```python
from build123d import *

# Parameters (mm, degrees)
SKETCH1_R           = 25
SKETCH1_W           = 27.8
SKETCH1_H           = 27.8
BOSS_EXTRUDE1_DEPTH = 55
BOSS_EXTRUDE2_START = 5
SKETCH2_R           = 25
SKETCH2_W           = 27.8
SKETCH2_H           = 27.8
BOSS_EXTRUDE2_DEPTH = 5
SKETCH3_W           = 25
SKETCH3_H           = 50
BOSS_EXTRUDE3_DEPTH = 80
FILLET1_R           = 2.5
FILLET2_R           = 2.5
SKETCH21_W          = 60
SKETCH21_H          = 20.6
CUT_EXTRUDE1_DEPTH  = 11.3
SKETCH22_W          = 40.5
SKETCH22_H          = 20.6
CUT_EXTRUDE2_DEPTH  = 93.059763198
CUT_EXTRUDE3_DEPTH  = 88.464278423
SKETCH23_R          = 2.15
CUT_EXTRUDE4_DEPTH  = 93.059763198
CUT_EXTRUDE7_DEPTH  = 27.5
CUT_EXTRUDE8_DEPTH  = 10


with BuildPart() as part:
    # Sketch1 → Boss-Extrude1 (new body)
    with BuildSketch(Plane.XY):
        Circle(SKETCH1_R)
        Rectangle(SKETCH1_W, SKETCH1_H, mode=Mode.SUBTRACT)
    extrude(amount=BOSS_EXTRUDE1_DEPTH)

    # Sketch2 → Boss-Extrude2 (add)
    # profile 1 of 2: a face of its own
    with BuildSketch(Plane(origin=(0, 0, 0), x_dir=(-1, 0, 0), z_dir=(0, 0, -1)).offset(BOSS_EXTRUDE2_START)):
        Circle(SKETCH2_R)
        Rectangle(SKETCH2_W, SKETCH2_H, mode=Mode.SUBTRACT)
    # profile 2 of 2: a face of its own
    with BuildSketch(Plane(origin=(0, 0, 0), x_dir=(-1, 0, 0), z_dir=(0, 0, -1)).offset(BOSS_EXTRUDE2_START)):
        Rectangle(SKETCH2_W, SKETCH2_H)
    extrude(amount=-BOSS_EXTRUDE2_DEPTH)

    # Sketch3 → Boss-Extrude3 (add)
    with BuildSketch(Plane(origin=(0, 0, -5), x_dir=(-1, 0, 0), z_dir=(0, 0, -1))):
        with Locations((12.5, 0)):
            Rectangle(SKETCH3_W, SKETCH3_H)
    extrude(amount=BOSS_EXTRUDE3_DEPTH)

    # Fillet1
    fillet1_edges = [part.edges().sort_by_distance(p)[0] for p in [
        (-13.9, 13.9, 27.5),
        (-13.9, -13.9, 27.5),
        (13.9, -13.9, 27.5),
        (13.9, 13.9, 27.5),
    ]]
    fillet(fillet1_edges, radius=FILLET1_R)

    # Fillet2
    fillet2_edges = [part.edges().sort_by_distance(p)[0] for p in [
        (0, 13.9, 55),
        (-13.9, 0, 55),
        (0, -13.9, 55),
        (13.9, 0, 55),
        (-13.167766953, 13.167766953, 55),
        (-13.167766953, -13.167766953, 55),
        (13.167766953, -13.167766953, 55),
        (13.167766953, 13.167766953, 55),
    ]]
    fillet(fillet2_edges, radius=FILLET2_R)

    # Sketch21 → Cut-Extrude1 (cut)
    with BuildSketch(Plane(origin=(0, 0, 0), x_dir=(0, 0, -1), z_dir=(1, 0, 0))):
        with Locations((52, 0)):
            Rectangle(SKETCH21_W, SKETCH21_H)
    extrude(amount=-CUT_EXTRUDE1_DEPTH, mode=Mode.SUBTRACT)

    # Sketch22 → Cut-Extrude2 (cut, through all)
    with BuildSketch(Plane(origin=(0, 0, 0), x_dir=(0, 0, -1), z_dir=(1, 0, 0))):
        with Locations((51.85, 0)):
            Rectangle(SKETCH22_W, SKETCH22_H)
    extrude(amount=-CUT_EXTRUDE2_DEPTH, mode=Mode.SUBTRACT)

    # Sketch18 → Cut-Extrude3 (cut, through all)
    with BuildSketch(Plane.XY.offset(-5)):
        with BuildLine():
            Line((-25, -25), (0, -25))
            ThreePointArc((0, -25), (-17.67766953, -17.67766953), (-25, 0))
            Line((-25, 0), (-25, -25))
        make_face()
        with BuildLine():
            Line((-25, 25), (-25, 0))
            ThreePointArc((-25, 0), (-17.67766953, 17.67766953), (0, 25))
            Line((0, 25), (-25, 25))
        make_face()
    extrude(amount=-CUT_EXTRUDE3_DEPTH, mode=Mode.SUBTRACT)

    # Sketch23 → Cut-Extrude4 (cut, through all)
    with BuildSketch(Plane(origin=(0, 0, 0), x_dir=(0, 0, -1), z_dir=(1, 0, 0))):
        with Locations(Location((27.85, -5.25, 0), (0, 0, 90))):
            Circle(SKETCH23_R)
        with Locations(Location((75.85, 5.25, 0), (0, 0, 90))):
            Circle(SKETCH23_R)
        with Locations(Location((75.85, -5.25, 0), (0, 0, 90))):
            Circle(SKETCH23_R)
        with Locations(Location((27.85, 5.25, 0), (0, 0, 90))):
            Circle(SKETCH23_R)
    extrude(amount=-CUT_EXTRUDE4_DEPTH, mode=Mode.SUBTRACT)

    # Sketch24 → Cut-Extrude7 (cut, symmetric)
    with BuildSketch(Plane(origin=(0, 0, -51.85), x_dir=(-1, 0, 0), z_dir=(0, 0, -1))):
        with BuildLine():
            Line((22.779596133, 10.3), (13.3, 10.3))
            Line((13.3, 10.3), (13.3, -10.3))
            Line((13.3, -10.3), (22.779596133, -10.3))
            ThreePointArc((22.779596133, -10.3), (25, 0), (22.779596133, 10.3))
        make_face()
    extrude(amount=CUT_EXTRUDE7_DEPTH, both=True, mode=Mode.SUBTRACT)

    # Sketch25 → Cut-Extrude8 (cut)
    with BuildSketch(Plane(origin=(0, 0, -24.35), x_dir=(-1, 0, 0), z_dir=(0, 0, -1))):
        with BuildLine():
            Line((13.3, -10.3), (22.779596133, -10.3))
            ThreePointArc((22.779596133, -10.3), (25, 0), (22.779596133, 10.3))
            Line((22.779596133, 10.3), (13.3, 10.3))
            Line((13.3, 10.3), (13.3, -10.3))
        make_face()
    extrude(amount=-CUT_EXTRUDE8_DEPTH, mode=Mode.SUBTRACT)


solid = part.part
```
Here's how the part is built. I have some questions about the finished solid (model axes, mm). A direction names the side the tool comes from. Coordinates: 2 decimals unless noted, no trailing zeros. Loops run counter-clockwise (first coordinate to the right, second up) from the corner with the lowest first, then second, coordinate; pieces in that order, holes last. Notation, with made-up numbers: M 34.25,14 L 68.25,14 A23 ccw 68.25,44 Z; hole C -17.75,57.25 d11. An arc over 180 degrees is marked long. One line per item, written item: value.
1. Imagine slicing it at D-D (x = 5). List the corners of the cut face in (y, z) for me, and give its area (3 significant figures).
Geometry says:
outline: M -24.49,-5 L 24.49,-5 L 24.49,55 L 16.4,55 A2.5 ccw 13.9,52.5 L 13.9,0 L -13.9,0 L -13.9,52.5 A2.5 ccw -16.4,55 L -24.49,55 Z
area: 1,410 mm2
2. Imagine slicing it at B-B (y = 5). State how many separate pieces and enclosed holes the cut face has, and give its area (3 significant figures).
Geometry says:
separate pieces: 4
enclosed holes: 0
area: 1,860 mm2
3. Imagine slicing it at A-A (z = -75.85). List the corners of the cut face in (x, y) for me, and give its area (3 significant figures).
Geometry says:
outline: M -22.78,-10.3 A25 ccw 0,-25 L 0,-10.3 L -11.3,-10.3 L -11.3,-7.4 L -13.3,-7.4 L -13.3,-10.3 Z; M -22.78,10.3 L -13.3,10.3 L -13.3,7.4 L -11.3,7.4 L -11.3,10.3 L 0,10.3 L 0,25 A25 ccw Z; M -13.3,-3.1 L -11.3,-3.1 L -11.3,3.1 L -13.3,3.1 Z
area: 506 mm2
4. Please list where these lines run through material, in increasing order: probe 1 along Z at (x, y) = (-12, -5); probe 2 along X at (y, z) = (0, 14); probe 3 along Z at (x, y) = (-22, -7).
Geometry says:
probe 1: z = -85 to -77.99, -73.71 to -72.1, -31.6 to -29.99, -25.71 to 0
probe 2: x = -25 to -13.9, 13.9 to 25
probe 3: z = -85 to -79.35, -14.35 to 55
5. Imagine slicing it at C-C (z = 46). List the corners of the cut face in (x, y) for me.
Geometry says:
outline: C 0,0 d50; hole M -13.9,-11.4 A2.5 ccw -11.4,-13.9 L 11.4,-13.9 A2.5 ccw 13.9,-11.4 L 13.9,11.4 A2.5 ccw 11.4,13.9 L -11.4,13.9 A2.5 ccw -13.9,11.4 Z
6. On a 3-axis mill with a long thin cutter (end or side, diameter ignored), from which of +Z, -Z, +X, -X, +Y, -Y can I reach the whole of each face in a straight line? I mean faces 3 (the cylindrical face through (-12.29, -5.72, -77.95)), 4 (the cylindrical face through (-13.187, -13.148, 26.618)), 5 (the flat face through (-13.3, 0, -76)), 6 (the flat face through (-11.3, 0, -77)). Say none if no direction works.
Geometry says:
face 3: +X, -X
face 4: +Z
face 5: -X
face 6: +X
7. Thinking about a two-plate mould opening in Y: for faces 1 (the cylindrical face through (13.148, 13.187, 26.618)), 2 (the flat face through (0, -11, -44)), which applies, +Y half, -Y half, draft (parallel to the pull), parting line (faces both ways), or undercut?
Geometry says:
face 1: undercut
face 2: draft
8. Will these pins go through, and if not, where does the flat tip stop? pin 1 Ø2 at (x, y) = (9, 12) entering from +Z; pin 2 Ø1.5 at (y, z) = (19, 24.5) entering from -X; pin 3 Ø12 at (x, z) = (-8.5, 27.5) entering from +Y; pin 4 Ø2 at (y, z) = (5, -27.5) entering from -X.
Geometry says:
pin 1: stops at z = 0
pin 2: stops at x = -17.09
pin 3: stops at y = 24.87
pin 4: passes through
